Input: part model. Units: mm. Frame: model coordinates. A direction names the side the tool comes from. Coordinates: 2 decimals unless noted, no trailing zeros. Loops run counter-clockwise (first coordinate to the right, second up) from the corner with the lowest first, then second, coordinate; pieces in that order, holes last.
```python
from build123d import *

# Parameters (mm, degrees)
CHANFREIN1_SIZE = 0.5
CONG_1_R        = 1.5
CHANFREIN2_SIZE = 0.2


with BuildPart() as part:
    # Esquisse1 → Base-Révolution (revolve)
    with BuildSketch(Plane.XY, mode=Mode.PRIVATE) as base_r_volution_sk:
        Polygon((60, 0), (60, -3), (50, -3), (50, -4), (0, -4), (0, -6.5), (-8, -6.5), (-8, 0), align=None)
    revolve(base_r_volution_sk.sketch.rotate(Axis((0, 0, 0), (1, 0, 0)), 270), axis=Axis((0, 0, 0), (1, 0, 0)))

    # Chanfrein1
    chanfrein1_edges = [part.edges().sort_by_distance(p)[0] for p in [
        (60, 0, -3),
    ]]
    chamfer(chanfrein1_edges, length=CHANFREIN1_SIZE)

    # Congé1
    cong_1_edges = [part.edges().sort_by_distance(p)[0] for p in [
        (-8, 0, -6.5),
    ]]
    fillet(cong_1_edges, radius=CONG_1_R)

    # Chanfrein2
    chanfrein2_edges = [part.edges().sort_by_distance(p)[0] for p in [
        (50, 0, -4),
    ]]
    chamfer(chanfrein2_edges, length=CHANFREIN2_SIZE)


solid = part.part
```
Item 1: Reachability of faces 1 (the face through (50, -1, -3)), 2 (the face through (60, 0, 0)) from +Z, -Z, +X, -X, +Y, -Y: full face, straight path, thin tool, end or side. Return the list, or none.
Result:
face 1: +X
face 2: +Z, -Z, +X, +Y, -Y
Item 2: Section query C-C (x = 17). Output: boundary loops of the cut face in (y, z).
Result:
outline: circle Ø8 at (0, 0)
Item 3: Contact query for flat-ended pins moving along their axis: P1, Ø6, axis at y = -3, z = 1.5, coming from the +X side; P2, Ø2, axis at x = 11.5, z = 1, coming from the +Y side; P3, Ø3, axis at x = 10.5, y = -3, coming from the -Z side; P4, Ø5, axis at x = 49.5, z = 0, coming from the -Y side. Output: stop coordinate, or through.
Result:
P1: stops at x = 60
P2: stops at y = 4
P3: stops at z = -3.71
P4: stops at y = -4
Item 4: Section query A-A (z = 0). Output: boundary loops of the cut face in (x, y), then the cut area to 3 significant figures.
Result:
outline: (-8, -5) arc R1.5 ccw to (-6.5, -6.5) - (0, -6.5) - (0, -4) - (49.8, -4) - (50, -3.8) - (50, -3) - (59.5, -3) - (60, -2.5) - (60, 2.5) - (59.5, 3) - (50, 3) - (50, 3.8) - (49.8, 4) - (0, 4) - (0, 6.5) - (-6.5, 6.5) arc R1.5 ccw to (-8, 5) - close
area: 563 mm2
Item 5: Line query: L1, parallel to X at y = -4.25, z = -3; L2, parallel to X at y = -1.5, z = -2.75; L3, parallel to Z at x = 32, y = 0.25. Output: solid intervals per line, ascending.
Result:
L1: x = -7.99 to 0
L2: x = -8 to 50
L3: z = -3.99 to 3.99
